Study the drawing (mm; zero at the part's minimum x, y, z) and answer. A direction names the side the tool comes from. Give positions to 0.01 mm unless a question says otherwise; leave off trailing zeros. Write each loop counter-clockwise with the first axis right and the second up, starting at its lowest first coordinate (ties: lowest second). Pieces come first, ordered by that corner, then holes.
1) Determine the mould class of the marked faces 3, 4 and 5 for opening direction X: pulls with the +X half, pulls with the -X half, needs draft (parallel to the pull), parting line crosses it, or undercut.
2) Find section C-C (y = 15). Determine the outline of the cut face in (x, z), plus the area to 3 significant figures.
3) Find section B-B (y = 37). Determine the outline of the cut face in (x, z).
4) Find section A-A (x = 3.5). Determine the outline of the cut face in (y, z), plus the area to 3 significant figures.
5) Straight lines are drawn through the part: probe 1 along X at (y, z) = (42, 9); probe 2 along Y at (x, z) = (10, 0.5); probe 3 along Y at (x, z) = (6.5, 8). For each, find the intervals that lie inside material, in ascending order.
6) A tool of negligible diameter and unlimited length cuts with its end or side. For the marked faces 1 and 2, from which of +Z, -Z, +X, -X, +Y, -Y can it reach the whole face along a straight path? Write none if from no direction.
7) Given pin 1 Ø4 at (x, z) = (12, 9) entering from -Y; pin 2 Ø5 at (x, y) = (6.5, 39.5) entering from +Z; pin 3 Ø5.5 at (x, y) = (8.5, 60.5) entering from +Z; pin 4 Ø3 at (x, z) = (8, 5) entering from -Y, each flat-ended and moving along its own axis, determine where each tip first touches the part or whether it passes through.
8) Find section D-D (z = 7.5). Determine the outline of the cut face in (x, y), plus the area to 3 significant figures.
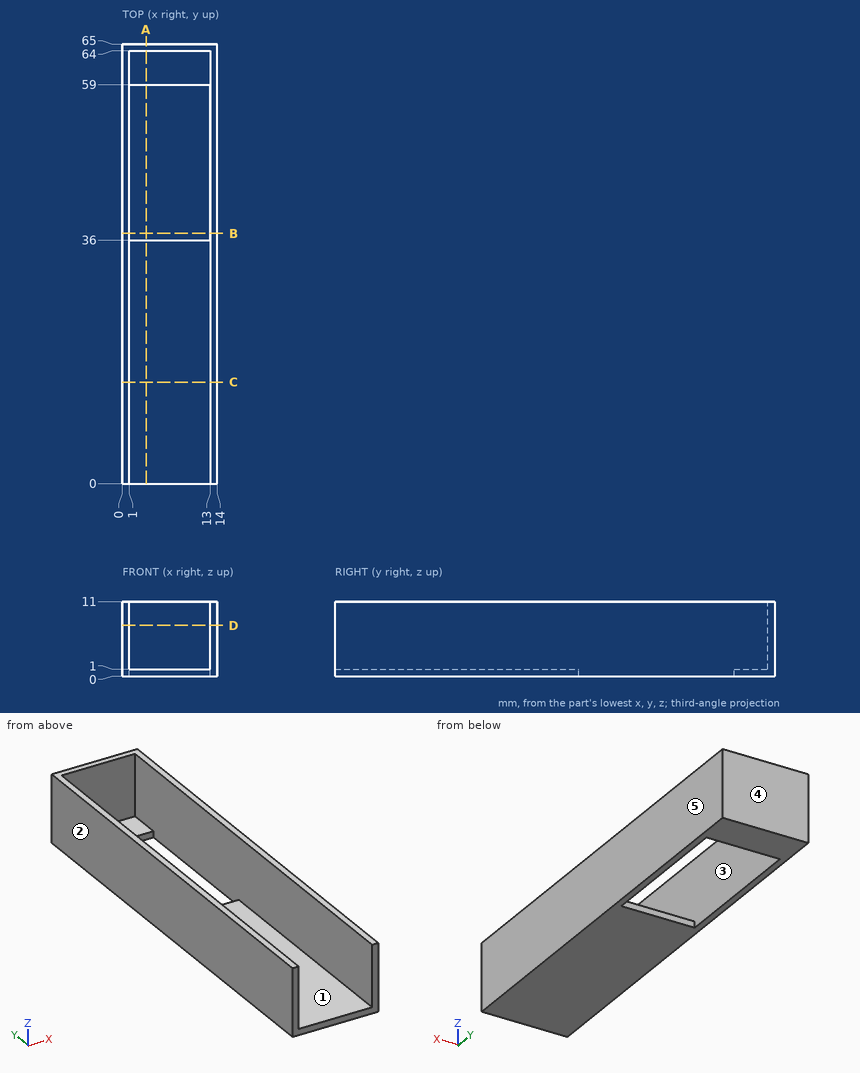
Results:
1. face 3: undercut
1. face 4: needs draft
1. face 5: pulls with the +X half
2. outline: (0, 0) - (14, 0) - (14, 11) - (13, 11) - (13, 1) - (1, 1) - (1, 11) - (0, 11) - close
2. area: 34.0 mm2
3. outline: (0, 0) - (1, 0) - (1, 11) - (0, 11) - close; (13, 0) - (14, 0) - (14, 11) - (13, 11) - close
4. outline: (0, 0) - (36, 0) - (36, 1) - (0, 1) - close; (59, 0) - (65, 0) - (65, 11) - (64, 11) - (64, 1) - (59, 1) - close
4. area: 52.0 mm2
5. probe 1: x = 0 to 1, 13 to 14
5. probe 2: y = 0 to 36, 59 to 65
5. probe 3: y = 64 to 65
6. face 1: +Z, -Y
6. face 2: +Z, -Z, -X, +Y, -Y
7. pin 1: stops at y = 0
7. pin 2: passes through
7. pin 3: stops at z = 1
7. pin 4: stops at y = 64
8. outline: (0, 0) - (1, 0) - (1, 64) - (13, 64) - (13, 0) - (14, 0) - (14, 65) - (0, 65) - close
8. area: 142 mm2
